Work out the finished part from the listing and answer in its coordinate system (mm). Give positions to 0.01 mm unless a question says otherwise; leave off trailing zeros. Loops run counter-clockwise (first coordinate to the right, second up) from the corner with the lowest first, then second, coordinate; pieces in that order, holes last. Notation, with made-up numbers: (31, 24) - (64, 24) arc R11 ccw to (64, 37) - close; hole circle Ø10 at (80, -35). An arc over 180 degrees is marked (long way). Use CSV: the item, a comma, the result in double quotes.
from build123d import *

# Parameters (mm, degrees)
SKETCH1_W                 = 76.2
SKETCH1_H                 = 25.4
SKETCH1_W_2               = 69.85
SKETCH1_H_2               = 19.05
BOSS_EXTRUDE1_DEPTH       = 427.2
FILLET1_R                 = 1
SKETCH2_R                 = 19
CUT_EXTRUDE1_DEPTH        = 430.647076099
F_4_0MM_DOWEL_HOLE1_D     = 4
F_4_0MM_DOWEL_HOLE2_D     = 4
F_4_0MM_DOWEL_HOLE2_DEPTH = 3.175


with BuildPart() as part:
    # Sketch1 → Boss-Extrude1 (new, symmetric)
    with BuildSketch(Plane(origin=(0, 0, 0), x_dir=(0, 0, -1), z_dir=(1, 0, 0))):
        Rectangle(SKETCH1_W, SKETCH1_H)
        Rectangle(SKETCH1_W_2, SKETCH1_H_2, mode=Mode.SUBTRACT)
    extrude(amount=BOSS_EXTRUDE1_DEPTH, both=True)

    # Fillet1
    fillet1_edges = [part.edges().sort_by_distance(p)[0] for p in [
        (0, 9.525, 34.925),
        (0, -9.525, 34.925),
        (0, -9.525, -34.925),
        (0, 9.525, -34.925),
        (0, 12.7, 38.1),
        (0, 12.7, -38.1),
        (0, -12.7, -38.1),
        (0, -12.7, 38.1),
    ]]
    fillet(fillet1_edges, radius=FILLET1_R)

    # Sketch2 → Cut-Extrude1 (cut, through all)
    with BuildSketch(Plane(origin=(0, 12.7, 0), x_dir=(1, 0, 0), z_dir=(0, 1, 0))):
        with Locations(Location((-152.4, 0, 0), (0, 0, 270))):
            Circle(SKETCH2_R)
    extrude(amount=-CUT_EXTRUDE1_DEPTH, mode=Mode.SUBTRACT)

    # Ø4.0mm Dowel Hole1 (through all)
    with Locations(Plane.XY.offset(38.1)):
        with Locations((-417.2, 0), (-397.2, 0)):
            f_4_0mm_dowel_hole1 = Hole(F_4_0MM_DOWEL_HOLE1_D / 2)

    # Mirror1: Ø4.0mm Dowel Hole1 across plane
    add(f_4_0mm_dowel_hole1.mirror(Plane(origin=(0, 0, 0), x_dir=(0, 0, 1), z_dir=(1, 0, 0))), mode=Mode.SUBTRACT)

    # Ø4.0mm Dowel Hole2
    with Locations(Plane(origin=(0, -12.7, 0), x_dir=(-1, 0, 0), z_dir=(0, -1, 0))):
        with Locations((180.96711396, -28.56711396), (180.96711396, 28.56711396), (123.83288604, 28.56711396), (123.83288604, -28.56711396)):
            Hole(F_4_0MM_DOWEL_HOLE2_D / 2, depth=F_4_0MM_DOWEL_HOLE2_DEPTH)


solid = part.part
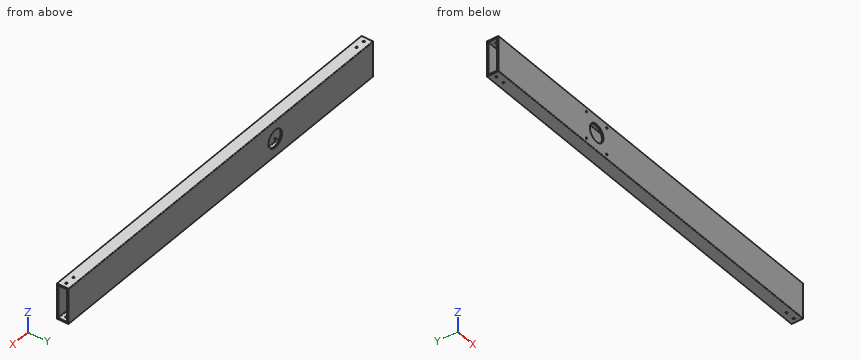
Item 1: A cutting plane is placed at B-B on x = -266.5. Determine the outline of the cut face in (y, z) (3 decimals).
Determined:
outline,"(-12.7, -37.1) arc R1 ccw to (-11.7, -38.1) - (11.7, -38.1) arc R1 ccw to (12.7, -37.1) - (12.7, 37.1) arc R1 ccw to (11.7, 38.1) - (-11.7, 38.1) arc R1 ccw to (-12.7, 37.1) - close; hole (-9.525, -33.925) arc R1 ccw to (-8.525, -34.925) - (8.525, -34.925) arc R1 ccw to (9.525, -33.925) - (9.525, 33.925) arc R1 ccw to (8.525, 34.925) - (-8.525, 34.925) arc R1 ccw to (-9.525, 33.925) - close"
Item 2: Given P1, Ø3, axis at x = -123.83, z = 28.57, coming from the -Y side (3 decimals), flat-ended and moving along its own axis, determine where the tip first touches the part or whether it passes through.
Determined:
P1,"stops at y = 9.525"
Item 3: Find the intervals of material crossed by line 1 (Y direction, x = 196.5, z = 2) (3 decimals); line 2 (Z direction, x = 64.5, y = -3.25) (3 decimals); line 3 (X direction, y = -10.6, z = 0), in increasing order.
Determined:
line 1,"y = -12.7 to -9.525, 9.525 to 12.7"
line 2,"z = -38.1 to -34.925, 34.925 to 38.1"
line 3,"x = -427.2 to -171.4, -133.4 to 427.2"
Item 4: A cutting plane is placed at A-A on z = 0. Determine the outline of the cut face in (x, y) (3 decimals).
Determined:
outline,"(-427.2, -12.7) - (-171.4, -12.7) - (-171.4, -9.525) - (-427.2, -9.525) - close; (-427.2, 9.525) - (-171.4, 9.525) - (-171.4, 12.7) - (-427.2, 12.7) - close; (-133.4, -12.7) - (427.2, -12.7) - (427.2, -9.525) - (-133.4, -9.525) - close; (-133.4, 9.525) - (427.2, 9.525) - (427.2, 12.7) - (-133.4, 12.7) - close"
